The model under review builds one solid part; all positions refer to its coordinate system, in mm. A direction names the side the tool comes from. Coordinates: 2 decimals unless noted, no trailing zeros. Order: outer loops, then holes, each group sorted by start corner. A loop starts at its lowest first (then second) coordinate and runs counter-clockwise, first axis right, second up.
Autodesk Inventor part; units mm, degrees
ref_plane "YZ Plane" through (0, 0, 0) normal (1, 0, 0) x (0, 1, 0)
ref_plane "XZ Plane" through (0, 0, 0) normal (0, 1, 0) x (-1, 0, 0)
ref_plane "XY Plane" through (0, 0, 0) normal (0, 0, 1) x (1, 0, 0)
sketch "Sketch_1" plane through (0, 0, 0) normal (0, 0, 1) x (1, 0, 0)
  line L0 (6, 0) -> (0, 0)
  line L1 (-0.8, 0) -> (-0.8, 2.7673)
  line L2 (-0.8, 2.7673) -> (-0.5333, 3.5)
  line L3 (-0.5333, 3.5) -> (0, 3.5)
  line L4 (0, 3.5) -> (0, 1.9)
  arc A0 (0, 1.9) -> (0.4, 1.5) centre (0.4, 1.9) ccw
  line L5 (0.4, 1.5) -> (6, 1.5)
  line L6 (6, 1.5) -> (6, 0)
  line L7 (6, 0) -> (-0.8, 0)
  line L8 (0, 0) -> (-0.8, 0)
  dimension "d6" = 6
revolve "Revolution1" add sketch "Sketch_1" angle 360 about axis through (6, 0, 0) along (1, 0, 0)
sketch "Sketch_5" plane through (-0.05, 0, 0) normal (1, 0, 0) x (0, 0, -1)
  arc A0 (-0.6801, -0.1159) -> (-0.4404, -0.531) centre (-0.5499, -0.3175) ccw
  arc A1 (-0.341, -0.5357) -> (-0.4404, -0.531) centre (-0.3947, -0.62) ccw
  arc A2 (-0.341, -0.5357) -> (-0.2934, -0.5632) centre (0, 0) ccw
  arc A3 (-0.2397, -0.6469) -> (-0.2934, -0.5632) centre (-0.3396, -0.6519) ccw
  arc A4 (-0.2397, -0.6469) -> (0.2397, -0.6469) centre (0, -0.635) ccw
  arc A5 (0.2934, -0.5632) -> (0.2397, -0.6469) centre (0.3396, -0.6519) ccw
  arc A6 (0.2934, -0.5632) -> (0.341, -0.5357) centre (0, 0) ccw
  arc A7 (0.4404, -0.531) -> (0.341, -0.5357) centre (0.3947, -0.62) ccw
  arc A8 (0.4404, -0.531) -> (0.6801, -0.1159) centre (0.5499, -0.3175) ccw
  arc A9 (0.6344, -0.0275) -> (0.6801, -0.1159) centre (0.7343, -0.0318) ccw
  arc A10 (0.6344, -0.0275) -> (0.6344, 0.0275) centre (0, 0) ccw
  arc A11 (0.6801, 0.1159) -> (0.6344, 0.0275) centre (0.7343, 0.0318) ccw
  arc A12 (0.6801, 0.1159) -> (0.4404, 0.531) centre (0.5499, 0.3175) ccw
  arc A13 (0.341, 0.5357) -> (0.4404, 0.531) centre (0.3947, 0.62) ccw
  arc A14 (0.341, 0.5357) -> (0.2934, 0.5632) centre (0, 0) ccw
  arc A15 (0.2397, 0.6469) -> (0.2934, 0.5632) centre (0.3396, 0.6519) ccw
  arc A16 (0.2397, 0.6469) -> (-0.2397, 0.6469) centre (0, 0.635) ccw
  arc A17 (-0.2934, 0.5632) -> (-0.2397, 0.6469) centre (-0.3396, 0.6519) ccw
  arc A18 (-0.2934, 0.5632) -> (-0.341, 0.5357) centre (0, 0) ccw
  arc A19 (-0.4404, 0.531) -> (-0.341, 0.5357) centre (-0.3947, 0.62) ccw
  arc A20 (-0.4404, 0.531) -> (-0.6801, 0.1159) centre (-0.5499, 0.3175) ccw
  arc A21 (-0.6344, 0.0275) -> (-0.6801, 0.1159) centre (-0.7343, 0.0318) ccw
  arc A22 (-0.6344, 0.0275) -> (-0.6344, -0.0275) centre (0, 0) ccw
  arc A23 (-0.6801, -0.1159) -> (-0.6344, -0.0275) centre (-0.7343, -0.0318) ccw
extrude "Extrusion1" cut sketch "Sketch_5" against normal blind 0.75
sketch "Sketch_2" plane through (0, 0, 0) normal (0, 0, 1) x (1, 0, 0)
  line L0 (0.4552, 0) -> (0, 0)
  line L1 (-0.05, 0) -> (-0.05, 0.875)
  line L2 (-0.05, 0.875) -> (0.4552, 0)
  line L3 (0.4552, 0) -> (-0.05, 0)
revolve "Revolution2" cut sketch "Sketch_2" angle 360 about axis through (0.4552, 0, 0) along (1, 0, 0)
sketch "スケッチ4" plane through (6, 0, 0) normal (1, 0, 0) x (0, 0, -1)
  circle A0 centre (0, 0) radius 1.5
extrude "押し出し2" add sketch "スケッチ4" along normal blind 4
thread "Thread1"
properties part number "超極低頭ネジL10" material "ステンレス鋼"
(1) Wall thickness on probe 1 along Y at (x, z) = (9.5, 0); probe 2 along X at (y, z) = (-2.5, -1); probe 3 along X at (y, z) = (2, -2.5): over which ranges is each line inside the solid? List them lowest first.
A:
probe 1: y = -1.5 to 1.5
probe 2: x = -0.8 to 0
probe 3: x = -0.64 to 0
(2) Machinability: for faces 4 (the face through (0, 2, -2)), 5 (the face through (-0.8, 0, 1)), which of the approach directions +Z, -Z, +X, -X, +Y, -Y give a long, thin tool a straight path to every point of the face, cutting with its end or side? Answer none if there is none.
A:
face 4: +X
face 5: +Z, -Z, -X, +Y, -Y
(3) Draft analysis for pull direction Z (two halves, no side actions). For faces 1 (the face through (-0.263, 3.233, -1.341)), 2 (the face through (0.367, -0.033, 0.148)), 3 (the face through (10, 0, 0)), state which applies: released by +Z, released by -Z, zero draft, split by the parting line, or undercut.
A:
face 1: split by the parting line
face 2: undercut
face 3: zero draft
(4) For pin 1 Ø1 at (y, z) = (2, -1.5) entering from +X; pin 2 Ø1.5 at (x, y) = (2, -0.5) entering from -Z; pin 3 Ø1 at (x, z) = (2, 1) entering from -Y, all flat-tipped, find the tip position at first contact; note any pin that passes through.
A:
pin 1: stops at x = 0
pin 2: stops at z = -1.5
pin 3: stops at y = -1.41
(5) We need section A-A, the plane x = 5. Write out the cut boundary in (y, z), and give its area (3 significant figures).
A:
outline: circle Ø3 at (0, 0)
area: 7.07 mm2
